Drawing for the job (mm, zero at the part's lowest x, y, z). A direction names the side the tool comes from. Give positions to 0.01 mm unless a question says otherwise; leave off trailing zeros. Order: outer loops, then holes, each group sorted by start corner. A loop starts at its lowest first (then second) coordinate and runs counter-clockwise, first axis right, second up. Notation, with made-up numbers: (28, 73) - (78, 73) arc R22 ccw to (78, 85) - close; hole circle Ø2 at (44.5, 13). An arc over 180 degrees is marked (long way). One line per item, written item: value.
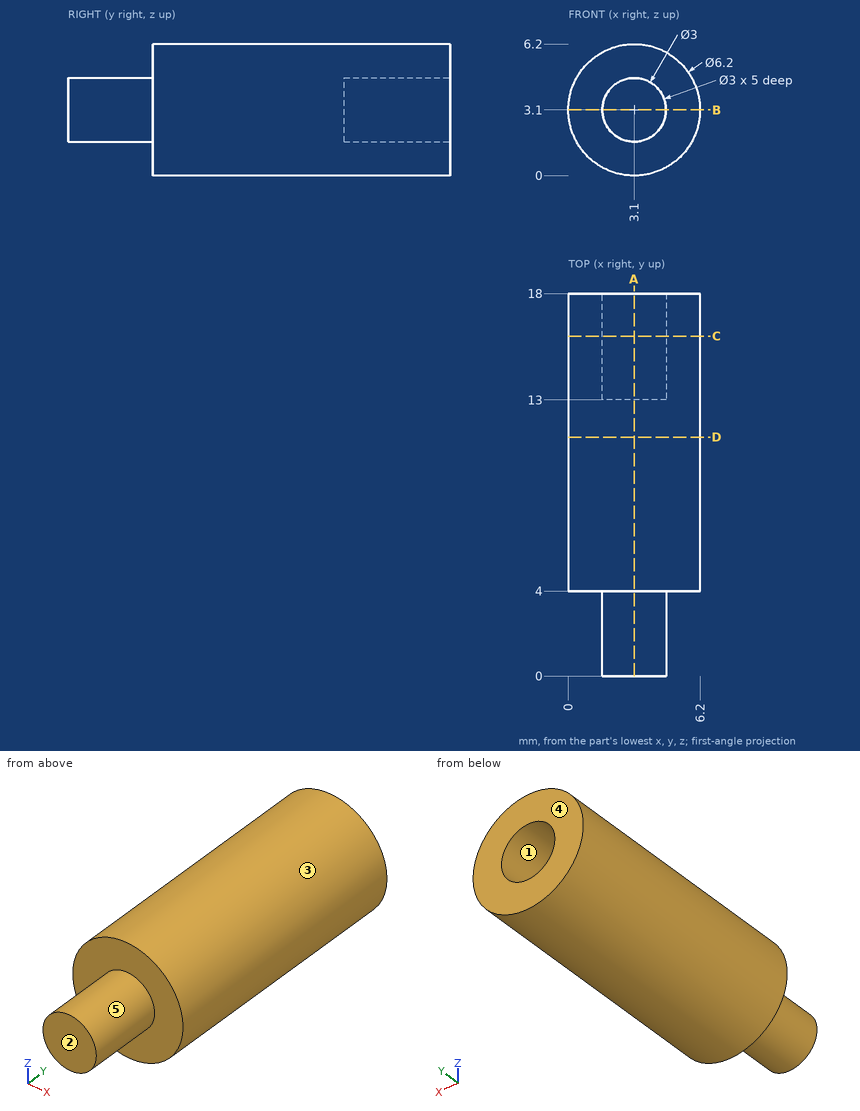
(1) 3-axis set-ups, long thin cutter, end or side, ignore diameter. For the marked faces 4 and 5: which of +Z, -Z, +X, -X, +Y, -Y reach the whole face in a straight line?
Completed:
face 4: +Z, -Z, +X, -X, +Y
face 5: -Y
(2) Pull direction Z, two halves, no side cores. Call the marked faces 1, 2 and 3: +Z half, -Z half, draft (parallel to the pull), parting line (faces both ways), or undercut.
Completed:
face 1: undercut
face 2: draft
face 3: parting line
(3) Pin check, flat tips, straight feed: P1, Ø1.5, axis at y = 15.5, z = 4, coming from the -X side; P2, Ø1, axis at y = 12.5, z = 4, coming from the +X side; P3, Ø1, axis at x = 5, y = 12, coming from the -Z side. Stop position of each tip, or through.
Completed:
P1: x = 0
P2: x = 6.17
P3: z = 0.33
(4) Slice it at D-D, the plane y = 11.25. Give the cut face in (x, z).
Completed:
outline: circle Ø6.2 at (3.1, 3.1)
(5) Drill centre lines: line 1 (X direction, y = 14.3, z = 3.1); line 2 (Y direction, x = 1.75, z = 1.5). Where is each one in solid material? Low to high.
Completed:
line 1: 0 to 1.6, 4.6 to 6.2
line 2: 4 to 18
(6) Slice it at C-C, the plane y = 16. Give the cut face in (x, z), and give its area (3 significant figures).
Completed:
outline: circle Ø6.2 at (3.1, 3.1); hole circle Ø3 at (3.1, 3.1)
area: 23.1 mm²
(7) Slice it at A-A, the plane x = 3.1. Give the cut face in (y, z).
Completed:
outline: (0, 1.6) - (4, 1.6) - (4, 0) - (18, 0) - (18, 1.6) - (13, 1.6) - (13, 4.6) - (18, 4.6) - (18, 6.2) - (4, 6.2) - (4, 4.6) - (0, 4.6) - close
(8) Slice it at B-B, the plane z = 3.1. Give the cut face in (x, y), and give its area (3 significant figures).
Completed:
outline: (0, 4) - (1.6, 4) - (1.6, 0) - (4.6, 0) - (4.6, 4) - (6.2, 4) - (6.2, 18) - (4.6, 18) - (4.6, 13) - (1.6, 13) - (1.6, 18) - (0, 18) - close
area: 83.8 mm²
